Build history of the part. All positions in model axes, mm. Round coordinates to 2 decimals unless told otherwise and drop trailing zeros. Loops run counter-clockwise (first coordinate to the right, second up) from the corner with the lowest first, then second, coordinate; pieces in that order, holes last.
from build123d import *

# Parameters (mm, degrees)
F1_DEPTH = 3


with BuildPart() as f1:
    # F0 (on Right) → F1 (new body)
    with BuildSketch(Plane.YZ):
        with BuildLine():
            Line((-33, 9), (-33, 0))
            Line((-33, 0), (-24, 0))
            ThreePointArc((-24, 0), (-26.6360389693, 6.3639610307), (-33, 9))
        make_face()
        with BuildLine():
            ThreePointArc((-37, 0), (-35, 2), (-33, 0))
            Line((-33, 0), (-33, 9))
            ThreePointArc((-33, 9), (-39.3639610307, 6.3639610307), (-42, 0))
            Line((-42, 0), (-37, 0))
        make_face()
        with BuildLine():
            Line((-24, 0), (-33, 0))
            Line((-33, 0), (-33, -9))
            ThreePointArc((-33, -9), (-26.6360389693, -6.3639610307), (-24, 0))
        make_face()
        with BuildLine():
            Line((-33, -9), (-33, 0))
            ThreePointArc((-33, 0), (-35, -2), (-37, 0))
            Line((-37, 0), (-42, 0))
            ThreePointArc((-42, 0), (-39.3639610307, -6.3639610307), (-33, -9))
        make_face()
        with BuildLine():
            ThreePointArc((-20, 0), (-22, -2), (-24, 0))
            ThreePointArc((-24, 0), (-26.6360389693, -6.3639610307), (-33, -9))
            Line((-33, -9), (-25, -9))
            Line((-25, -9), (-4.3588989435, -9))
            ThreePointArc((-4.3588989435, -9), (-8.4731632061, -5.310885546), (-10, 0))
            Line((-10, 0), (-20, 0))
        make_face()
        with BuildLine():
            ThreePointArc((-33, 9), (-26.6360389693, 6.3639610307), (-24, 0))
            ThreePointArc((-24, 0), (-22, 2), (-20, 0))
            Line((-20, 0), (-10, 0))
            ThreePointArc((-10, 0), (-7.0710678119, 7.0710678119), (0, 10))
            Line((0, 10), (0, 20))
            ThreePointArc((0, 20), (-2, 21.9999999928), (-1.44e-08, 24))
            ThreePointArc((-1.44e-08, 24), (-4.7434164964, 25.3514707334), (-8.0622577483, 29))
            Line((-8.0622577483, 29), (-9, 29))
            Line((-9, 29), (-9, 25))
            ThreePointArc((-9, 25), (-13.686291501, 13.686291501), (-25, 9))
            Line((-25, 9), (-33, 9))
        make_face()
        with BuildLine():
            ThreePointArc((-42, 0), (-39.3639610307, 6.3639610307), (-33, 9))
            Line((-33, 9), (-25, 9))
            ThreePointArc((-25, 9), (-13.686291501, 13.686291501), (-9, 25))
            Line((-9, 25), (-9, 29))
            Line((-9, 29), (-42, 29))
            Line((-42, 29), (-42, 0))
        make_face()
        with BuildLine():
            Line((-42, -9), (-33, -9))
            ThreePointArc((-33, -9), (-39.3639610307, -6.3639610307), (-42, 0))
            Line((-42, 0), (-42, -9))
        make_face()
        with BuildLine():
            ThreePointArc((0, 10), (-7.0710678119, 7.0710678119), (-10, 0))
            Line((-10, 0), (-6, 0))
            ThreePointArc((-6, 0), (-4.2426406871, 4.2426406871), (0, 6))
            Line((0, 6), (0, 10))
        make_face()
        with BuildLine():
            Line((-6, 0), (-10, 0))
            ThreePointArc((-10, 0), (-8.4731632061, -5.310885546), (-4.3588989435, -9))
            Line((-4.3588989435, -9), (0, -9))
            Line((0, -9), (0, -6))
            ThreePointArc((0, -6), (-4.2426406871, -4.2426406871), (-6, 0))
        make_face()
        with BuildLine():
            Line((-42, 34), (-42, 29))
            Line((-42, 29), (-9, 29))
            Line((-9, 29), (-9, 33))
            ThreePointArc((-9, 33), (-8.9860571774, 33.5007758031), (-8.94427191, 34))
            Line((-8.94427191, 34), (-42, 34))
        make_face()
        with BuildLine():
            ThreePointArc((10, 0), (7.0710678119, 7.0710678119), (0, 10))
            Line((0, 10), (0, 6))
            ThreePointArc((0, 6), (4.2426406871, 4.2426406871), (6, 0))
            Line((6, 0), (10, 0))
        make_face()
        with BuildLine():
            Line((0, 20), (0, 10))
            ThreePointArc((0, 10), (7.0710678119, 7.0710678119), (10, 0))
            Line((10, 0), (20, 0))
            ThreePointArc((20, 0), (22, 2), (24, 0))
            ThreePointArc((24, 0), (26.6360389693, 6.3639610307), (33, 9))
            Line((33, 9), (25, 9))
            ThreePointArc((25, 9), (13.686291501, 13.686291501), (9, 25))
            Line((9, 25), (9, 29))
            Line((9, 29), (8.0622577483, 29))
            ThreePointArc((8.0622577483, 29), (4.7434164841, 25.3514707258), (-1.44e-08, 24))
            ThreePointArc((-1.44e-08, 24), (1.4142135573, 23.4142135675), (2, 22))
            ThreePointArc((2, 22), (1.4142135624, 20.5857864376), (0, 20))
        make_face()
        with BuildLine():
            Line((-9, 33), (-9, 29))
            Line((-9, 29), (-8.0622577483, 29))
            ThreePointArc((-8.0622577483, 29), (-8.7624288794, 30.9457750531), (-9, 33))
        make_face()
        with BuildLine():
            Line((0, -6), (0, -9))
            Line((0, -9), (4.3588989435, -9))
            ThreePointArc((4.3588989435, -9), (8.4731632061, -5.310885546), (10, 0))
            Line((10, 0), (6, 0))
            ThreePointArc((6, 0), (4.2426406871, -4.2426406871), (0, -6))
        make_face()
        with BuildLine():
            Line((20, 0), (10, 0))
            ThreePointArc((10, 0), (8.4731632061, -5.310885546), (4.3588989435, -9))
            Line((4.3588989435, -9), (25, -9))
            Line((25, -9), (33, -9))
            ThreePointArc((33, -9), (26.6360389693, -6.3639610307), (24, 0))
            ThreePointArc((24, 0), (22, -2), (20, 0))
        make_face()
        with BuildLine():
            Line((0, 33), (-9, 33))
            ThreePointArc((-9, 33), (-8.7624288794, 30.9457750531), (-8.0622577483, 29))
            Line((-8.0622577483, 29), (0, 29))
            Line((0, 29), (0, 33))
        make_face()
        with BuildLine():
            ThreePointArc((-8.94427191, 34), (-8.9860571774, 33.5007758031), (-9, 33))
            Line((-9, 33), (0, 33))
            ThreePointArc((0, 33), (-1, 33.2679491924), (-1.7320508076, 34))
            Line((-1.7320508076, 34), (-8.94427191, 34))
        make_face()
        with BuildLine():
            Line((0, 29), (-8.0622577483, 29))
            ThreePointArc((-8.0622577483, 29), (-4.7434164964, 25.3514707334), (-1.44e-08, 24))
            Line((0, 24), (0, 29))
        make_face()
        with BuildLine():
            Line((0, 29), (0, 24))
            ThreePointArc((-1.44e-08, 24), (4.7434164841, 25.3514707258), (8.0622577483, 29))
            Line((8.0622577483, 29), (0, 29))
        make_face()
        with BuildLine():
            ThreePointArc((-1.7320508076, 34), (-1, 33.2679491924), (0, 33))
            Line((0, 33), (0, 34))
            Line((0, 34), (-1.7320508076, 34))
        make_face()
        with BuildLine():
            ThreePointArc((1.7320508076, 34), (1, 33.2679491924), (0, 33))
            Line((0, 33), (0, 29))
            Line((0, 29), (8.0622577483, 29))
            ThreePointArc((8.0622577483, 29), (8.7624288794, 30.9457750531), (9, 33))
            ThreePointArc((9, 33), (8.9860571774, 33.5007758031), (8.94427191, 34))
            Line((8.94427191, 34), (1.7320508076, 34))
        make_face()
        with BuildLine():
            Line((0, 34), (0, 33))
            ThreePointArc((0, 33), (1, 33.2679491924), (1.7320508076, 34))
            Line((1.7320508076, 34), (0, 34))
        make_face()
        with BuildLine():
            ThreePointArc((9, 33), (8.7624288794, 30.9457750531), (8.0622577483, 29))
            Line((8.0622577483, 29), (9, 29))
            Line((9, 29), (9, 33))
        make_face()
        with BuildLine():
            ThreePointArc((33, 9), (26.6360389693, 6.3639610307), (24, 0))
            Line((24, 0), (33, 0))
            ThreePointArc((33, 0), (35, 2), (37, 0))
            Line((37, 0), (42, 0))
            ThreePointArc((42, 0), (39.3639610307, 6.3639610307), (33, 9))
        make_face()
        with BuildLine():
            Line((33, 0), (24, 0))
            ThreePointArc((24, 0), (26.6360389693, -6.3639610307), (33, -9))
            Line((33, -9), (33, 0))
        make_face()
        with BuildLine():
            Line((42, 34), (8.94427191, 34))
            ThreePointArc((8.94427191, 34), (8.9860571774, 33.5007758031), (9, 33))
            Line((9, 33), (9, 29))
            Line((9, 29), (42, 29))
            Line((42, 29), (42, 34))
        make_face()
        with BuildLine():
            Line((33, 0), (33, -9))
            ThreePointArc((33, -9), (39.3639610307, -6.3639610307), (42, 0))
            Line((42, 0), (37, 0))
            ThreePointArc((37, 0), (35, -2), (33, 0))
        make_face()
        with BuildLine():
            ThreePointArc((42, 0), (39.3639610307, -6.3639610307), (33, -9))
            Line((33, -9), (42, -9))
            Line((42, -9), (42, 0))
        make_face()
        with BuildLine():
            Line((42, 29), (9, 29))
            Line((9, 29), (9, 25))
            ThreePointArc((9, 25), (13.686291501, 13.686291501), (25, 9))
            Line((25, 9), (33, 9))
            ThreePointArc((33, 9), (39.3639610307, 6.3639610307), (42, 0))
            Line((42, 0), (42, 29))
        make_face()
    extrude(amount=F1_DEPTH)


solid = f1.part
(1) Probe line 1 (Z direction, x = 1.6, y = -35); line 2 (Y direction, x = 1.6, z = 21). List the from-to ranges inside material, lowest first.
Responses:
line 1: z = -9 to -2, 2 to 34
line 2: y = -42 to -1.73, 1.73 to 42
(2) Slice it at B-B on x = 1.1. List the corners of the cut face in (y, z), plus the area to 3 significant figures.
Responses:
outline: (-42, -9) - (42, -9) - (42, 34) - (-42, 34) - close; hole circle Ø4 at (-35, 0); hole circle Ø4 at (-22, 0); hole circle Ø12 at (0, 0); hole circle Ø4 at (0, 22); hole circle Ø4 at (22, 0); hole circle Ø4 at (35, 0)
area: 3,440 mm2
(3) Pull direction Y, two halves, no side cores. Call faces 1 (the face through (0, -1, 13)), 2 (the face through (1, 42, 12)), 3 (the face through (1.5, 20.4, 1.2)): +Y half, -Y half, draft (parallel to the pull), parting line (faces both ways), or undercut.
Responses:
face 1: draft
face 2: +Y half
face 3: undercut
(4) Slice it at A-A on y = 35. List the corners of the cut face in (x, z).
Responses:
outline: (0, -9) - (3, -9) - (3, -2) - (0, -2) - close; (0, 2) - (3, 2) - (3, 34) - (0, 34) - close
